```python
from build123d import *

# Parameters (mm, degrees)
BOTTOM_CENTER_CASING_DEPTH = 1.51892
SKETCH3_W                  = 76.2
SKETCH3_H                  = 1.51892
BOSS_EXTRUDE1_DEPTH        = 25.4
SKETCH4_R                  = 6.35
CUT_EXTRUDE1_DEPTH         = 25.4


with BuildPart() as part:
    # Sketch1 → Bottom Center Casing (new body)
    with BuildSketch(Plane.XY):
        with BuildLine():
            Line((-152.4, 100), (-15, 100))
            ThreePointArc((-15, 100), (0, 85), (15, 100))
            Line((15, 100), (152.4, 100))
            Line((152.4, 100), (152.4, -100))
            Line((152.4, -100), (-152.4, -100))
            Line((-152.4, -100), (-152.4, 100))
        make_face()
    extrude(amount=BOTTOM_CENTER_CASING_DEPTH)

    # Sketch3 → Boss-Extrude1 (add)
    with BuildSketch(Plane.XY.offset(1.51892)):
        with Locations((-114.3, 99.24054)):
            Rectangle(SKETCH3_W, SKETCH3_H)
        with Locations((114.3, 99.24054)):
            Rectangle(SKETCH3_W, SKETCH3_H)
    extrude(amount=BOSS_EXTRUDE1_DEPTH)

    # Sketch4 → Cut-Extrude1 (cut)
    with BuildSketch(Plane(origin=(0, 100, 0), x_dir=(1, 0, 0), z_dir=(0, 1, 0))):
        with Locations((-133.35, -13.649325)):
            Circle(SKETCH4_R)
        with Locations((-95.25, -14.029055)):
            Circle(SKETCH4_R)
        with Locations((95.25, -14.029055)):
            Circle(SKETCH4_R)
        with Locations((133.35, -13.649325)):
            Circle(SKETCH4_R)
    extrude(amount=-CUT_EXTRUDE1_DEPTH, mode=Mode.SUBTRACT)


solid = part.part
```
Part model, mm, in its own coordinate system. A direction names the side the tool comes from. Coordinates: 2 decimals unless noted, no trailing zeros. Order: outer loops, then holes, each group sorted by start corner. A loop starts at its lowest first (then second) coordinate and runs counter-clockwise, first axis right, second up. Notation, with made-up numbers: (61, -18.5) -> (90, -18.5) arc R25 ccw to (90, -4.5) -> close; hole circle Ø7 at (73, 1). An arc over 180 degrees is marked (long way). Put each result on its own line as item: value. Start each with the question number.
(1) Band-saw the part on D-D (x = -24.5). Give the cut face in (y, z).
(2) Mould opens along Z. For faces 3 (the face through (-127.293, 99.251, 11.742)), 4 (the face through (-152.4, -0.5, 0.4)), 5 (the face through (2, 1, 0)) say: pulls with the +Z half, pulls with the -Z half, needs draft (parallel to the pull), parting line crosses it, or undercut.
(3) Band-saw the part on C-C (y = -62.5). Give the cut face in (x, z).
(4) Pin check, flat tips, straight feed: pin 1 Ø10 at (x, z) = (133.35, 13.65) entering from -Y; pin 2 Ø8 at (x, y) = (68, -47.5) entering from +Z; pin 3 Ø10 at (y, z) = (-66, 4) entering from -X; pin 4 Ø10 at (x, z) = (-119.5, 19) entering from -Y. Stop position of each tip, or through.
(5) Band-saw the part on A-A (x = -133.35). Give the cut face in (y, z), then the cut area to 3 significant figures.
(6) Probe line 1 along Z through (x, y) = (-133.35, 99.65); line 2 along Z through (x, y) = (95.25, 99.25); line 3 along Z through (x, y) = (-112, -45). List the from-to ranges inside material, lowest first. Write a range as [from, to].
(7) Which spindle directions (+Z, -Z, +X, -X, +Y, -Y) get a long thin tool onto all of the face, cutting with end or side? Do faces 1 (the face through (114, 98.481, 14)), 2 (the face through (101.3, 99.3, 12.1)). Say none if no direction does.
(8) Band-saw the part on B-B (x = 121.5). Give the cut face in (y, z), then the cut area to 3 significant figures.
Determined:
1. outline: (-100, 0) -> (100, 0) -> (100, 1.52) -> (-100, 1.52) -> close
2. face 3: undercut
2. face 4: needs draft
2. face 5: pulls with the -Z half
3. outline: (-152.4, 0) -> (152.4, 0) -> (152.4, 1.52) -> (-152.4, 1.52) -> close
4. pin 1: passes through
4. pin 2: stops at z = 1.52
4. pin 3: stops at x = -152.4
4. pin 4: stops at y = 98.48
5. outline: (-100, 0) -> (100, 0) -> (100, 7.3) -> (98.48, 7.3) -> (98.48, 1.52) -> (-100, 1.52) -> close; (98.48, 20) -> (100, 20) -> (100, 26.92) -> (98.48, 26.92) -> close
5. area: 323 mm²
6. line 1: z = [0, 7.3], [20, 26.92]
6. line 2: z = [0, 7.68], [20.38, 26.92]
6. line 3: z = [0, 1.52]
7. face 1: +Z, +X, -X, -Y
7. face 2: +Y, -Y
8. outline: (-100, 0) -> (100, 0) -> (100, 26.92) -> (98.48, 26.92) -> (98.48, 1.52) -> (-100, 1.52) -> close
8. area: 342 mm²
